```python
from build123d import *

# Parameters (mm, degrees)
CUT_EXTRUDE1_REACH = 62.854


with BuildPart() as part:
    # Sketch3 → Revolve1 (revolve)
    with BuildSketch(Plane.XY, mode=Mode.PRIVATE) as revolve1_sk:
        with BuildLine():
            Line((0, 0), (0, 17.9))
            Line((0, 17.9), (10, 17.9))
            Line((10, 17.9), (10, 19))
            Line((10, 19), (48, 19))
            Line((48, 19), (48, 17.9))
            Line((48, 17.9), (51, 17.9))
            ThreePointArc((51, 17.9), (52.414213562, 17.314213562), (53, 15.9))
            Line((53, 15.9), (53, 5))
            Line((53, 5), (57, 5))
            Line((57, 5), (57, 1.6))
            Line((57, 1.6), (64.6, 1.6))
            Line((64.6, 1.6), (64.6, 0))
            Line((64.6, 0), (49.67547572, 0))
            Line((49.67547572, 0), (49.67547572, 14.100571752))
            Line((49.67547572, 14.100571752), (3.511968533, 14.100571752))
            Line((3.511968533, 14.100571752), (3.511968533, 0))
            Line((3.511968533, 0), (0, 0))
        make_face()
    revolve(revolve1_sk.sketch.rotate(Axis((0, 0, 0), (1, 0, 0)), 90), axis=Axis((0, 0, 0), (1, 0, 0)))

    # Sketch4 → Cut-Extrude1 (cut, up to next)
    with BuildSketch(Plane.ZY.offset(-10), mode=Mode.PRIVATE) as cut_extrude1_sk1:
        with BuildLine():
            Line((1.5875, 18.933563947), (1.5875, 17.829465605))
            ThreePointArc((1.5875, 17.829465605), (0, 17.9), (-1.5875, 17.829465605))
            Line((-1.5875, 17.829465605), (-1.5875, 18.933563947))
            ThreePointArc((-1.5875, 18.933563947), (0, 19), (1.5875, 18.933563947))
        make_face()
    cut_extrude1_tool1 = extrude(cut_extrude1_sk1.sketch, amount=-CUT_EXTRUDE1_REACH, mode=Mode.PRIVATE) & part.part
    add(cut_extrude1_tool1.solids().sort_by_distance((10, 18.427166, 0))[0], mode=Mode.SUBTRACT)


solid = part.part
```
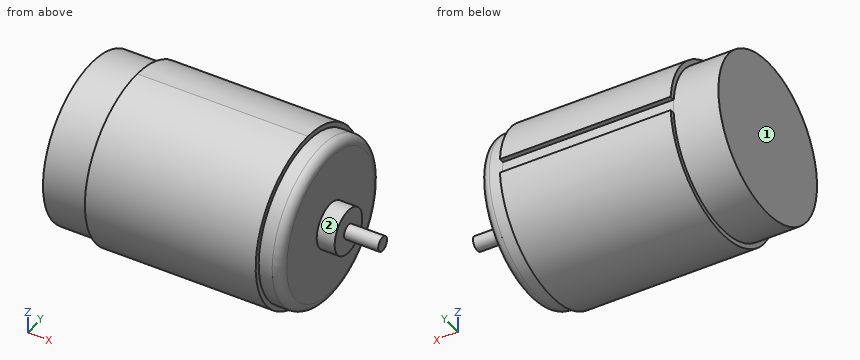
Check sheet for the modelled part. Datum: model origin and axes. Units: mm. Face numbers are marked on the shaded views. A direction names the side the tool comes from. Give positions to 0.01 mm unless a question says otherwise; leave off trailing zeros. Loops run counter-clockwise (first coordinate to the right, second up) from the corner with the lowest first, then second, coordinate; pieces in that order, holes last. Notation, with made-up numbers: (4, 45.5) - (54, 45.5) arc R19 ccw to (54, 74.5) - close; hole circle Ø11 at (40.25, -38). An arc over 180 degrees is marked (long way). One line per question, with ' | ' between items. Start each with the question number.
1. Cross-section at C-C, the plane x = 58. Enter the section's corners in (y, z).
2. Material ranges on line 1 along Y through (x, z) = (33, 0); line 2 along X through (y, z) = (-4, -1); line 3 along X through (y, z) = (3.5, 6), recorded low to high. Write a range as [from, to].
3. Gauge pin test, flat ends, axial feed: pin 1 Ø3 at (y, z) = (-14, 13.5) entering from -X; pin 2 Ø2 at (y, z) = (-5, 11) entering from +X; pin 3 Ø1 at (x, y) = (45, 1.5) entering from -Z. Record the tip position at first contact, or that the pin passes through.
4. Cross-section at B-B, the plane z = 0. Enter the section's corners in (x, y), plus the area to 3 significant figures.
5. Set-up check for the marked faces 1 and 2: record each of +Z, -Z, +X, -X, +Y, -Y from which the full face is reachable in a straight line by a thin tool's end or side.
6. Cross-section at A-A, the plane x = 28. Enter the section's corners in (y, z), plus the area to 3 significant figures.
Check result:
1) outline: circle Ø3.2 at (0, 0)
2) line 1: y = [-19, -14.1], [14.1, 17.9] | line 2: x = [0, 3.51], [49.68, 57] | line 3: x = [0, 3.51], [49.68, 53]
3) pin 1: stops at x = 10 | pin 2: stops at x = 53 | pin 3: stops at z = -18.97
4) outline: (0, -17.9) - (10, -17.9) - (10, -19) - (48, -19) - (48, -17.9) - (51, -17.9) arc R2 ccw to (53, -15.9) - (53, -5) - (57, -5) - (57, -1.6) - (64.6, -1.6) - (64.6, 1.6) - (57, 1.6) - (57, 5) - (53, 5) - (53, 15.9) arc R2 ccw to (51, 17.9) - (0, 17.9) - close; hole (3.51, -14.1) - (49.68, -14.1) - (49.68, 14.1) - (3.51, 14.1) - close | area: 700 mm2
5) face 1: +Z, -Z, -X, +Y, -Y | face 2: +X
6) outline: (17.83, -1.59) arc R17.9 ccw to (17.83, 1.59) - (18.93, 1.59) arc R19 ccw (long way) to (18.93, -1.59) - close; hole circle Ø28.2 at (0, 0) | area: 506 mm2
